from build123d import *

# Parameters (mm, degrees)
SCHIZZO1_W                      = 300
SCHIZZO1_H                      = 20
ESTRUSIONE_ESTRUSIONE1_DEPTH    = 10
FORO_FILETTATO_M6_5_D           = 5
FORO_FILETTATO_M6_5_CSINK_D     = 6
FORO_FILETTATO_M6_5_CSINK_ANGLE = 90
RACCORDO1_R                     = 5


with BuildPart() as part:
    # Schizzo1 → Estrusione-Estrusione1 (new body)
    with BuildSketch(Plane(origin=(0, 0, 0), x_dir=(1, 0, 0), z_dir=(0, 1, 0))):
        Rectangle(SCHIZZO1_W, SCHIZZO1_H)
    extrude(amount=ESTRUSIONE_ESTRUSIONE1_DEPTH)

    # Foro filettato M6-5 (through all)
    with Locations(Plane(origin=(0, 10, 0), x_dir=(1, 0, 0), z_dir=(0, 1, 0))):
        with Locations((-140, 0), (140, 0)):
            CounterSinkHole(FORO_FILETTATO_M6_5_D / 2, FORO_FILETTATO_M6_5_CSINK_D / 2, counter_sink_angle=FORO_FILETTATO_M6_5_CSINK_ANGLE)

    # Raccordo1
    raccordo1_edges = [part.edges().sort_by_distance(p)[0] for p in [
        (150, 5, 10),
        (-150, 5, 10),
        (-150, 5, -10),
        (150, 5, -10),
    ]]
    fillet(raccordo1_edges, radius=RACCORDO1_R)


solid = part.part
Source: CAD feature listing. Evaluate the final solid. Frame: model axes, mm. Round coordinates to 2 decimals unless told otherwise and drop trailing zeros. Loops run counter-clockwise (first coordinate to the right, second up) from the corner with the lowest first, then second, coordinate; pieces in that order, holes last. Notation, with made-up numbers: M 84,44 L 117,44 A32 cw 117,72 Z; hole C 15.5,54.5 d8. An arc over 180 degrees is marked long. Return JSON: item names as keys, results as strings. Group by question number.
1. Pin query (flat end, axial travel): pin 1 (4.5 mm diameter, centred on x = -140, z = 0, fed in from +Y); pin 2 (1 mm diameter, centred on y = 2.5, z = 6, fed in from -X). Return the tip coordinate at first contact, or that it passes through.
2. Mould query, pull axis X, two halves, no side actions, for faces 1 (the face through (137.615, 4.684, -0.751)), 2 (the face through (150, 5, 0)), 3 (the face through (-2, 0, 0)). Classes: released by +X, released by -X, zero draft, split by the parting line, or undercut.
3. Section query B-B on z = 0. Output: boundary loops of the cut face in (x, y), and give its area (3 significant figures).
4. Material intervals for line 1 along Z through (x, y) = (-140, 2); line 2 along X through (y, z) = (1.75, -2.25); line 3 along X through (y, z) = (3.75, 1.25), sorted ascending. Write a range as from..to.
5. Section query A-A on x = 140. Output: boundary loops of the cut face in (y, z).
Checks:
{
 "1": {"pin 1": "passes through", "pin 2": "stops at x = -149.97"},
 "2": {"face 1": "undercut", "face 2": "released by +X", "face 3": "zero draft"},
 "3": {"outline": "M -150,0 L -142.5,0 L -142.5,9.5 L -143,10 L -150,10 Z; M -137.5,0 L 137.5,0 L 137.5,9.5 L 137,10 L -137,10 L -137.5,9.5 Z; M 142.5,0 L 150,0 L 150,10 L 143,10 L 142.5,9.5 Z", "area": "2,900 mm²"},
 "4": {"line 1": "z = -10..-2.5, 2.5..10", "line 2": "x = -150..-141.09, -138.91..138.91, 141.09..150", "line 3": "x = -150..-142.17, -137.83..137.83, 142.17..150"},
 "5": {"outline": "M 0,-10 L 10,-10 L 10,-3 L 9.5,-2.5 L 0,-2.5 Z; M 0,2.5 L 9.5,2.5 L 10,3 L 10,10 L 0,10 Z"}
}
